Design review of the part built by this model. Coordinates are the model's own, in mm. Face numbers are marked on the shaded views. Round coordinates to 2 decimals unless told otherwise and drop trailing zeros. Order: outer loops, then holes, each group sorted by start corner. A loop starts at its lowest first (then second) coordinate and runs counter-clockwise, first axis right, second up. Notation, with made-up numbers: M -1,-38 L 34,-38 A20 cw 34,-24 Z; hole C 84,51 d6. An arc over 180 degrees is marked long. Write each question's results on one line, items separated by ' | '. Start each with the question number.
Item 1: Clearance check with a flat-ended pin moving along its axis: pin 1 (4 mm diameter, centred on x = 0, z = 0, fed in from +Y). State where the tip first meets the part, or that it passes through.
Item 2: Wall thickness on line 1 (X direction, y = -0.1, z = 0); line 2 (Z direction, x = 13.5, y = 0.3); line 3 (X direction, y = 0.15, z = 1.5): over which ranges is each line inside the solid? List them lowest first. Write a range as [from, to].
Item 3: Take a section at A-A, the plane z = 0. Write out the cut boundary in (x, y), plus the area to 3 significant figures.
Item 4: Take a section at B-B, the plane y = 0.2. Write out the cut boundary in (x, z).
Item 5: The part is to be moulded in two halves that separate along Z. For the marked faces 1, 2 and 3, say which applies: +Z half, -Z half, draft (parallel to the pull), parting line (faces both ways), or undercut.
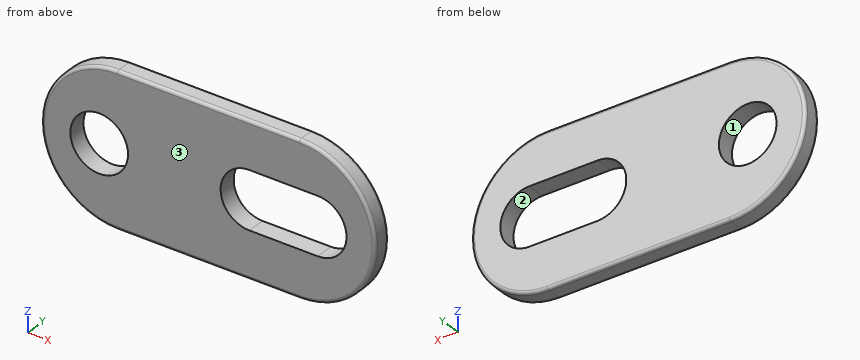
```python
from build123d import *

# Parameters (mm, degrees)
SKETCH1_R      = 2.413
EXTRUDE1_DEPTH = 0.762
FILLET1_R      = 0.254


with BuildPart() as part:
    # Sketch1 → Extrude1 (new body, symmetric)
    with BuildSketch(Plane(origin=(0, 0, 0), x_dir=(1, 0, 0), z_dir=(0, 1, 0))):
        with BuildLine():
            Line((1.524, -6.35), (16.764, -6.35))
            ThreePointArc((16.764, -6.35), (23.114, 0), (16.764, 6.35))
            Line((16.764, 6.35), (1.524, 6.35))
            ThreePointArc((1.524, 6.35), (-4.826, 0), (1.524, -6.35))
        make_face()
        Circle(SKETCH1_R, mode=Mode.SUBTRACT)
        with BuildLine():
            Line((12.573, 2.413), (18.288, 2.413))
            ThreePointArc((18.288, 2.413), (20.701, 0), (18.288, -2.413))
            Line((18.288, -2.413), (12.573, -2.413))
            ThreePointArc((12.573, -2.413), (10.16, 0), (12.573, 2.413))
        make_face(mode=Mode.SUBTRACT)
    extrude(amount=EXTRUDE1_DEPTH, both=True)

    # Fillet1
    fillet1_edges = [part.edges().sort_by_distance(p)[0] for p in [
        (23.114, 0.762, 0),
        (9.144, 0.762, -6.35),
        (-4.826, 0.762, 0),
        (9.144, -0.762, -6.35),
        (23.114, -0.762, 0),
        (9.144, -0.762, 6.35),
        (-4.826, -0.762, 0),
        (9.144, 0.762, 6.35),
    ]]
    fillet(fillet1_edges, radius=FILLET1_R)


solid = part.part
```
Results list:
1) pin 1: through
2) line 1: [-4.83, -2.41], [2.41, 10.16], [20.7, 23.11] | line 2: [-6.35, -2.41], [2.41, 6.35] | line 3: [-4.65, -1.89], [1.89, 10.68], [20.18, 22.93]
3) outline: M -4.83,-0.51 A0.25 ccw -4.57,-0.76 L -2.41,-0.76 L -2.41,0.76 L -4.57,0.76 A0.25 ccw -4.83,0.51 Z; M 2.41,-0.76 L 10.16,-0.76 L 10.16,0.76 L 2.41,0.76 Z; M 20.7,-0.76 L 22.86,-0.76 A0.25 ccw 23.11,-0.51 L 23.11,0.51 A0.25 ccw 22.86,0.76 L 20.7,0.76 Z | area: 19.1 mm²
4) outline: M 1.52,-6.35 L 16.76,-6.35 A6.35 ccw 16.76,6.35 L 1.52,6.35 A6.35 ccw Z; hole C 0,0 d4.83; hole M 12.57,-2.41 L 18.29,-2.41 A2.41 ccw 18.29,2.41 L 12.57,2.41 A2.41 ccw Z
5) face 1: undercut | face 2: undercut | face 3: draft
